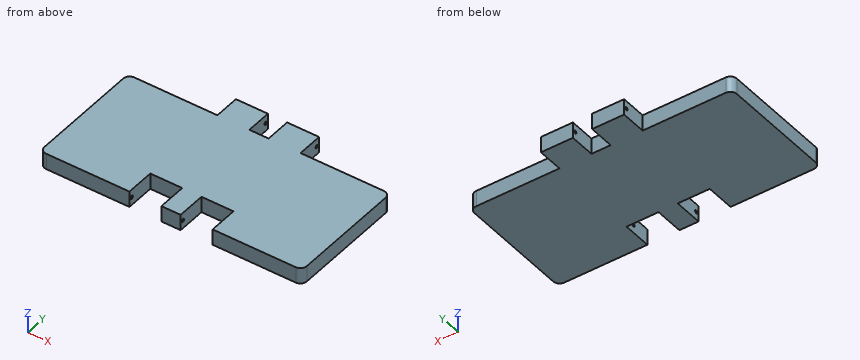
```python
from build123d import *

# Parameters (mm, degrees)
F1_DEPTH  = 5
F2_R      = 0.5
F3_DEPTH  = 2
F4_R      = 0.5
F5_DEPTH  = 5
F6_R      = 0.5
F7_DEPTH  = 2
F8_R      = 0.5
F9_DEPTH  = 5
F10_R     = 0.5
F11_DEPTH = 14.478


with BuildPart() as f1:
    # F0 (on Top) → F1 (new body)
    with BuildSketch(Plane.XY):
        with BuildLine():
            ThreePointArc((-39, 19), (-40.4142135624, 18.4142135624), (-41, 17))
            Line((-41, 17), (-41, -17))
            ThreePointArc((-41, -17), (-40.4142135624, -18.4142135624), (-39, -19))
            Line((-39, -19), (-13, -19))
            Line((-13, -19), (-13, -10))
            Line((-13, -10), (-3, -10))
            Line((-3, -10), (-3, -19))
            Line((-3, -19), (3, -19))
            Line((3, -19), (3, -10))
            Line((3, -10), (13, -10))
            Line((13, -10), (13, -19))
            Line((13, -19), (39, -19))
            ThreePointArc((39, -19), (40.4142135624, -18.4142135624), (41, -17))
            Line((41, -17), (41, 17))
            ThreePointArc((41, 17), (40.4142135624, 18.4142135624), (39, 19))
            Line((39, 19), (13, 19))
            Line((13, 19), (13, 27))
            Line((13, 27), (3, 27))
            Line((3, 27), (3, 19))
            Line((3, 19), (-3, 19))
            Line((-3, 19), (-3, 27))
            Line((-3, 27), (-13, 27))
            Line((-13, 27), (-13, 19))
            Line((-13, 19), (-39, 19))
        make_face()
    extrude(amount=F1_DEPTH)

    # F2 (on face) → F3 (cut)
    with BuildSketch(Plane.YZ.offset(3)):
        with Locations((-18, 2.5)):
            Circle(F2_R)
    extrude(amount=-F3_DEPTH, mode=Mode.SUBTRACT)

    # F4 (on face) → F5 (cut)
    with BuildSketch(Plane(origin=(13, 0, 0), x_dir=(0, -1, 0), z_dir=(-1, 0, 0))):
        with Locations((13, 2.5)):
            Circle(F4_R)
    extrude(amount=-F5_DEPTH, mode=Mode.SUBTRACT)

    # F6 (on face) → F7 (cut)
    with BuildSketch(Plane(origin=(-3, 0, 0), x_dir=(0, -1, 0), z_dir=(-1, 0, 0))):
        with Locations((18, 2.5)):
            Circle(F6_R)
    extrude(amount=-F7_DEPTH, mode=Mode.SUBTRACT)

    # F8 (on face) → F9 (cut)
    with BuildSketch(Plane.YZ.offset(-13)):
        with Locations((-18, 2.5)):
            Circle(F8_R)
    extrude(amount=-F9_DEPTH, mode=Mode.SUBTRACT)

    # F10 (on Right) → F11 (cut, symmetric)
    with BuildSketch(Plane.YZ):
        with Locations((26, 2.5)):
            Circle(F10_R)
    extrude(amount=F11_DEPTH, both=True, mode=Mode.SUBTRACT)


solid = f1.part
```
The listing builds one solid part. Answer for the finished solid, in the listing's coordinates (mm). Round coordinates to 2 decimals unless told otherwise and drop trailing zeros. Loops run counter-clockwise (first coordinate to the right, second up) from the corner with the lowest first, then second, coordinate; pieces in that order, holes last. Notation, with made-up numbers: (-17, -31.75) -> (37, -31.75) arc R7 ccw to (37, -23.75) -> close; hole circle Ø10 at (88, -32.75). An arc over 180 degrees is marked (long way). Use one line per item in the form item = value.
1. The part is cut by section B-B on x = 4. Determine the outline of the cut face in (y, z), and give its area (3 significant figures).
Answer key:
outline = (-10, 0) -> (27, 0) -> (27, 5) -> (-10, 5) -> close; hole circle Ø1 at (26, 2.5)
area = 184 mm²
2. Flat-ended cylindrical pins translate along their axes: pin 1 Ø1.5 at (x, z) = (-9, 2.5) entering from -Y; pin 2 Ø2.5 at (y, z) = (21.5, 3.5) entering from +X; pin 3 Ø3 at (x, y) = (-0.5, 2) entering from -Z; pin 4 Ø1.1 at (y, z) = (-18, 2.5) entering from -X. Find the tip coordinate at first contact, or state that the pin passes through.
Answer key:
pin_1 = -10
pin_2 = 13
pin_3 = 0
pin_4 = -40.95
3. The part is cut by section C-C on z = 3.9. Determine the outline of the cut face in (x, y), and give its area (3 significant figures).
Answer key:
outline = (-41, -17) arc R2 ccw to (-39, -19) -> (-13, -19) -> (-13, -10) -> (-3, -10) -> (-3, -19) -> (3, -19) -> (3, -10) -> (13, -10) -> (13, -19) -> (39, -19) arc R2 ccw to (41, -17) -> (41, 17) arc R2 ccw to (39, 19) -> (13, 19) -> (13, 27) -> (3, 27) -> (3, 19) -> (-3, 19) -> (-3, 27) -> (-13, 27) -> (-13, 19) -> (-39, 19) arc R2 ccw to (-41, 17) -> close
area = 3,090 mm²
4. The part is cut by section A-A on y = -11.5. Determine the outline of the cut face in (x, z), and give its area (3 significant figures).
Answer key:
outline = (-41, 0) -> (-13, 0) -> (-13, 5) -> (-41, 5) -> close; (-3, 0) -> (3, 0) -> (3, 5) -> (-3, 5) -> close; (13, 0) -> (41, 0) -> (41, 5) -> (13, 5) -> close
area = 310 mm²
5. Find the intervals of material crossed by probe 1 along X at (y, z) = (-10.5, 3.45); probe 2 along X at (y, z) = (22.5, 2.95); probe 3 along Z at (x, y) = (2, -18), in increasing order. Write a range as [from, to].
Answer key:
probe_1 = [-41, -13], [-3, 3], [13, 41]
probe_2 = [-13, -3], [3, 13]
probe_3 = [0, 2], [3, 5]
6. The part is cut by section D-D on x = -36. Determine the outline of the cut face in (y, z).
Answer key:
outline = (-19, 0) -> (19, 0) -> (19, 5) -> (-19, 5) -> close
